Check sheet for the drawn part. Datum: minimum x, y, z corner. Units: mm. A direction names the side the tool comes from. Coordinates: 2 decimals unless noted, no trailing zeros. Loops run counter-clockwise (first coordinate to the right, second up) from the corner with the lowest first, then second, coordinate; pieces in that order, holes last.
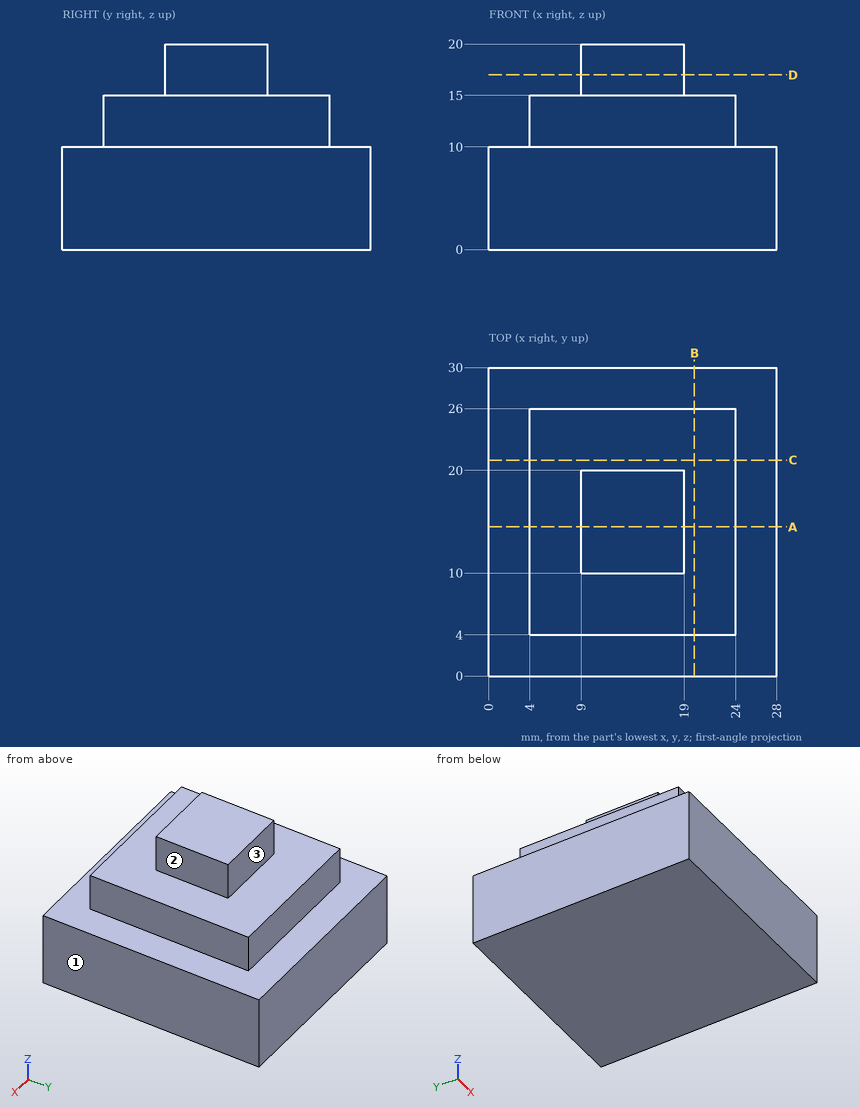
1) Scan lines: line 1 (Z direction, x = 19.5, y = 12.5); line 2 (X direction, y = 16.5, z = 13); line 3 (Z direction, x = 13.25, y = 2). Record each from-to range of solid material in increasing order.
Answer sheet:
line 1: z = 0 to 15
line 2: x = 4 to 24
line 3: z = 0 to 10
2) Section check A-A on y = 14.5. Enter the section's corners in (x, z), plus the area to 3 significant figures.
Answer sheet:
outline: (0, 0) - (28, 0) - (28, 10) - (24, 10) - (24, 15) - (19, 15) - (19, 20) - (9, 20) - (9, 15) - (4, 15) - (4, 10) - (0, 10) - close
area: 430 mm2
3) Set-up check for the marked faces 1, 2 and 3: record each of +Z, -Z, +X, -X, +Y, -Y from which the full face is reachable in a straight line by a thin tool's end or side.
Answer sheet:
face 1: +Z, -Z, +X, +Y, -Y
face 2: +Z, +X, +Y, -Y
face 3: +Z, +X, -X, +Y
4) Section check D-D on z = 17. Enter the section's corners in (x, y).
Answer sheet:
outline: (9, 10) - (19, 10) - (19, 20) - (9, 20) - close
5) Section check C-C on y = 21. Enter the section's corners in (x, z).
Answer sheet:
outline: (0, 0) - (28, 0) - (28, 10) - (24, 10) - (24, 15) - (4, 15) - (4, 10) - (0, 10) - close
6) Section check B-B on x = 20. Enter the section's corners in (y, z), plus the area to 3 significant figures.
Answer sheet:
outline: (0, 0) - (30, 0) - (30, 10) - (26, 10) - (26, 15) - (4, 15) - (4, 10) - (0, 10) - close
area: 410 mm2
7) Depth check by flat-ended pin: pin 1 (4 mm diameter, centred on y = 13.5, z = 13, fed in from +X); pin 2 (10 mm diameter, centred on x = 16, z = 17.5, fed in from +Y); pin 3 (2.5 mm diameter, centred on y = 16, z = 13, fed in from -X). Enter the tip coordinate at first touch or a pass-through.
Answer sheet:
pin 1: stops at x = 24
pin 2: stops at y = 26
pin 3: stops at x = 4
